Geometry: see drawing. Coordinates: mm, zero at the bounding-box minimum. Give positions to 0.01 mm unless a question says otherwise; leave off trailing zeros. Order: outer loops, then holes, each group sorted by start corner. A loop starts at its lowest first (then second) coordinate and runs counter-clockwise, first axis right, second up. Notation, with made-up numbers: (77, 43) - (87, 43) arc R25 ccw to (87, 57) - close; hole circle Ø8 at (-11.75, 49.25). An arc over 180 degrees is marked (long way). One line per item, written item: value.
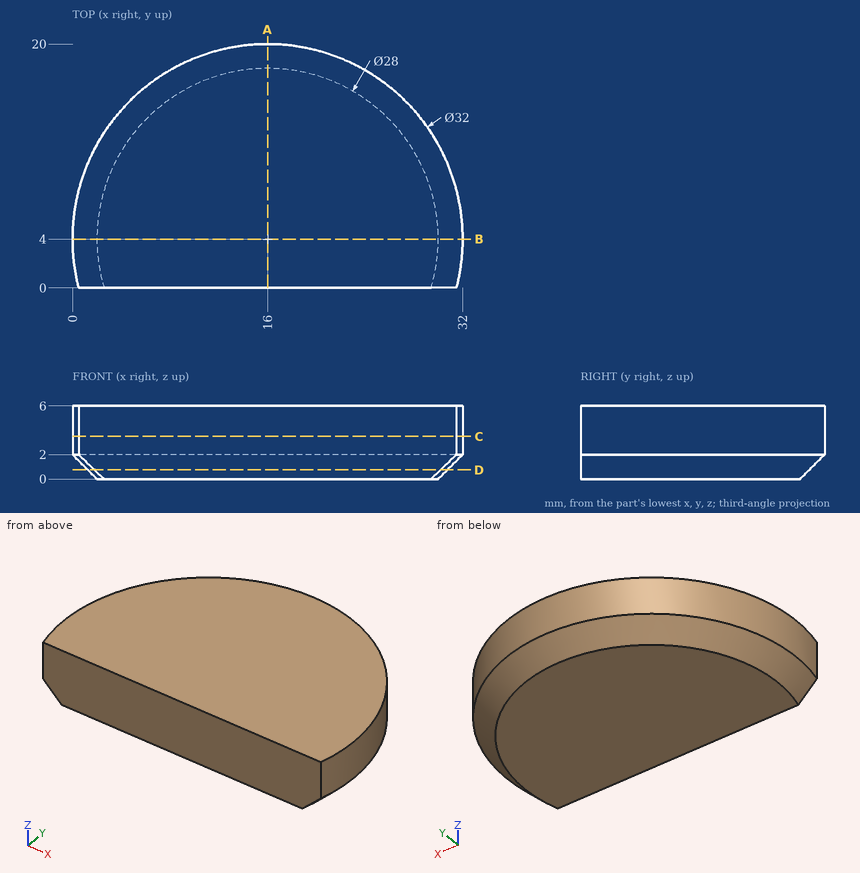
1) Material intervals for line 1 along X through (y, z) = (3.75, 3.5); line 2 along Y through (x, z) = (28, 5.5); line 3 along Y through (x, z) = (8, 5.5), sorted ascending.
Answers below:
line 1: 0 to 32
line 2: 0 to 14.58
line 3: 0 to 17.86
2) Section C-C, the plane z = 3.5. Return loops of the section in (x, y), then the cut area to 3 significant figures.
Answers below:
outline: (0.51, 0) - (31.49, 0) arc R16 ccw (long way) to start
area: 529 mm^2
3) First-contact query: pin 1 (1.5 mm diameter, centred on y = 9.5, z = 4.5, fed in from -X); pin 2 (2 mm diameter, centred on x = 25, z = 4.5, fed in from +Y). Flat tips, straight axial feed; report the tip coordinate or a pass-through.
Answers below:
pin 1: x = 0.72
pin 2: y = 17.86
4) Section A-A, the plane x = 16. Return loops of the section in (y, z).
Answers below:
outline: (0, 0) - (18, 0) - (20, 2) - (20, 6) - (0, 6) - close
5) Section D-D, the plane z = 0.75. Return loops of the section in (x, y), then the cut area to 3 significant figures.
Answers below:
outline: (1.8, 0) - (30.2, 0) arc R14.75 ccw (long way) to start
area: 458 mm^2
6) Section B-B, the plane y = 4. Return loops of the section in (x, z).
Answers below:
outline: (0, 2) - (2, 0) - (30, 0) - (32, 2) - (32, 6) - (0, 6) - close
